Could you check a few things on this model? Use its own coordinates, in mm. Face numbers are marked on the shaded views. A direction names the side the tool comes from. Coordinates: 2 decimals unless noted, no trailing zeros. Loops run counter-clockwise (first coordinate to the right, second up) from the corner with the lowest first, then second, coordinate; pieces in that order, holes last. Notation, with made-up numbers: M 17.25,39 L 24.25,39 A8 ccw 24.25,53 Z; hole C 33.25,-27.5 d2. An arc over 180 degrees is marked long. Write each question's results on one line, items separated by ' | '.
Autodesk Inventor part; units mm, degrees
ref_plane "Work Plane1" through (52.845, 0, 0) normal (0, 0, -1) x (-1, 0, 0)
ref_plane "YZ Plane" through (0, 0, 0) normal (1, 0, 0) x (0, 1, 0)
ref_plane "XZ Plane" through (0, 0, 0) normal (0, 1, 0) x (-1, 0, 0)
sketch "Schizzo1" plane through (0, 0, 0) normal (0, 0, 1) x (1, 0, 0)
  line L0 (-4.5484, 0) -> (24.4414, 0)
  line L1 (6.3771, 12) -> (4.5751, 15.8643)
  line L2 (6.3771, 12) -> (20.3, 12) construction
  line L3 (20.3, 12) -> (20.3, 0) construction
  arc A0 (4.5751, 15.8643) -> (0, 14.85) centre (2.4, 14.85) ccw
  line L4 (6.3771, 12) -> (6.3771, 0)
  line L5 (0, -3.5401) -> (0, 21.2403)
  point P0 (0, 0)
  dimension "d1" = 24
  dimension "d3" = 34.5
  dimension "d4" = 2.4
  dimension "d16" = 20.3
  dimension "d17" = 25
revolve "Anello" add sketch "Schizzo1" angle 360 about axis through (-10, 0, 0) along (1, 0, 0)
sketch "Schizzo2" plane through (0, 0, 0) normal (-1, 0, 0) x (0, 0, 1)
  circle A0 centre (0, 0) radius 4.9
  line L0 (-12, -6.9282) -> (-12, 6.9282)
  line L1 (-12, 6.9282) -> (0, 13.8564)
  line L2 (0, 13.8564) -> (12, 6.9282)
  line L3 (12, 6.9282) -> (12, -6.9282)
  line L4 (12, -6.9282) -> (0, -13.8564)
  line L5 (0, -13.8564) -> (-12, -6.9282)
  circle A1 centre (0, 0) radius 14.85
  dimension "d5" = 27.7128
extrude "Corpo" add sketch "Schizzo2" against normal blind 15.3 contours A0 | L0 L1 L2 L3 L4 L5
sketch "Schizzo3" plane through (15.3, 0, 0) normal (1, 0, 0) x (0, 0, -1)
  circle A0 centre (0, 0) radius 12
  dimension "d19" = 24
extrude "Corona" add sketch "Schizzo3" along normal blind 5
sketch "Schizzo4" plane through (0, 0, 0) normal (-1, 0, 0) x (0, 0, 1)
  circle A0 centre (0, 0) radius 4.9
  circle A1 centre (0, 0) radius 14.85
hole "Filettatura" at (0, 0, 0) direction (1, 0, 0) diameter 13.835 end through all
sketch "Schizzo5" plane through (0, 0, 0) normal (0, 0, 1) x (1, 0, 0)
  line L0 (5.5114, 13.8564) -> (15.3, 13.8564)
  line L1 (15.3, 6.9282) -> (15.3, 13.8564)
  line L2 (0, -14.85) -> (0, 14.85)
  line L3 (-3.06, 0) -> (18.36, 0)
  line L4 (14.2282, 13.8564) -> (15.3, 12)
  dimension "d9" = 30
  dimension "d10" = 24
revolve "Smusso1" cut sketch "Schizzo5" angle 360 about axis through (-10, 0, 0) along (1, 0, 0)
chamfer "Smusso2" distance 1.0825 angle 30 1 edges at (0, 0, -6.9175) measured on face at (0, 12.0452, -1.4626)
ref_plane "Work Plane1" through (52.845, 0, 0) normal (0, 0, -1) x (-1, 0, 0)
equation "\"d1\" = SW"
equation "\"d3\" = LADI"
equation "\"d4\" = PHH"
equation "\"d16\" = KOH"
equation "\"d17\" = KEWI"
equation "\"d5\" = 1.1547 * SW"
equation "\"d6\" = KOH1"
equation "\"d19\" = SD2"
equation "\"d11\" = KOH - KOH1"
equation "\"d9\" = ANG1"
equation "\"d10\" = SW0"
equation "\"d13\" = -0.5 * GD1 + 0.5 * NND"
equation "\"d57\" = -0.5 * GD1 + 0.5 * NND"
equation "\"ANG1\" = 30deg"
equation "\"KEWI\" = 25deg"
equation "\"NND\" = 16"
equation "\"LADI\" = 34.5"
equation "\"SW\" = 24"
equation "\"PHH\" = 2.4"
equation "\"KOH\" = 20.3"
equation "\"SW0\" = SW"
equation "\"d0\" = LADI"
equation "\"d2\" = PHH"
equation "\"KOH1\" = 15.3"
equation "\"SD2\" = SW"
equation "\"GUL\" = 0.541266 * PTC"
equation "\"RR\" = PHH"
equation "\"THREADDIA\" = 16"
equation "\"TOA\" = 30deg"
equation "\"PTC\" = 2"
equation "\"GAL\" = 0.541266 * PTC"
equation "\"E0\" = 1.155 * SW"
properties part number "ISO 7043 - M16" material "Acciaio"
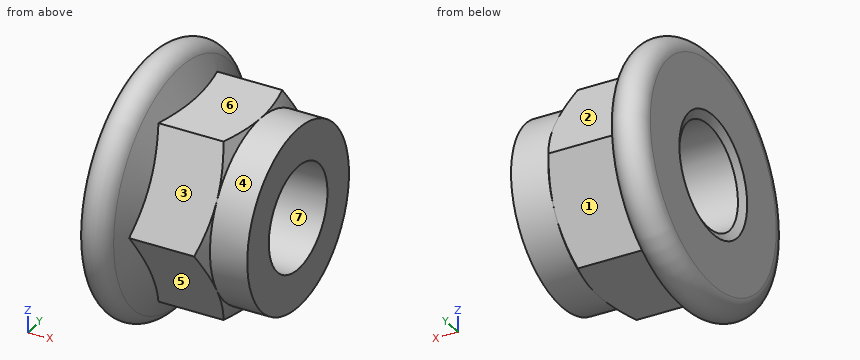
(1) If we mould it in two halves opening along Z, with no side actions, what happens to the marked faces 5, 6 and 7? For each: released by +Z, released by -Z, zero draft, split by the parting line, or undercut.
Reported:
face 5: released by -Z | face 6: released by +Z | face 7: undercut
(2) Imagine slicing it at A-A, the plane x = 8. List the corners of the cut face in (y, z) for me (1 decimal).
Reported:
outline: M -13.9,0 L -6.9,-12 L 6.9,-12 L 13.9,0 L 6.9,12 L -6.9,12 Z; hole C 0,0 d13.8
(3) Will these pins go through, and if not, where does the flat tip stop? P1, Ø10, axis at x = 14, y = 7.5, coming from the -Z side; P2, Ø2, axis at x = 18, y = -4.5, coming from the +Z side; P3, Ø8, axis at x = 9.5, y = 0, coming from the +Z side.
Reported:
P1: stops at z = -12 | P2: stops at z = 11.48 | P3: stops at z = 13.88
(4) Which directions (+Z, -Z, +X, -X, +Y, -Y) give clear straight access to the entire face, cutting with the end or side of a thin tool? Please do the marked faces 1, 2, 3 and 4.
Reported:
face 1: -Z, +X, +Y | face 2: +Z, +X, +Y | face 3: +Z, +X, -Y | face 4: +X
(5) Please list where these lines run through material, in increasing order: probe 1 along Y at (x, z) = (9, 0); probe 2 along Z at (x, y) = (1.5, -1); probe 3 along Z at (x, y) = (15.75, 0). Write a range as from..to.
Reported:
probe 1: y = -13.86..-6.92, 6.92..13.86 | probe 2: z = -17.05..-6.84, 6.84..17.05 | probe 3: z = -12..-6.92, 6.92..12
